Input: part model. Units: mm. Frame: model coordinates. A direction names the side the tool comes from. Round coordinates to 2 decimals unless told otherwise and drop trailing zeros. Loops run counter-clockwise (first coordinate to the right, second up) from the corner with the lowest first, then second, coordinate; pieces in that order, holes last.
(1) Cut plane A-A, the plane x = 0. Output: boundary loops of the cut face in (y, z).
(2) Cut plane B-B, the plane y = 0.75. Output: boundary loops of the cut face in (x, z).
(3) Access query for faces 1 (the face through (-1.245, 3.95, -3.002)), 2 (the face through (2, 2, 1)), 3 (the face through (-0.03, 0.27, -1.73)). Directions: +Z, -Z, +X, -X, +Y, -Y. A direction counts if a zero-diameter tool reaches every point of the face in a straight line with its end or side. Return the directions, or none.
(4) Draft query along Z for faces 4 (the face through (2, 3.2, 0)), 5 (the face through (0, 0, -2.3)), 6 (the face through (0.05, 0.13, -2.92)). Return one class per face: released by +Z, released by -Z, zero draft, split by the parting line, or undercut.
(5) Cut plane D-D, the plane y = 5.75. Output: boundary loops of the cut face in (x, z), and give its area (3 significant figures).
(6) Cut plane C-C, the plane z = 0. Output: boundary loops of the cut face in (x, y), and give its area (3 significant figures).
(7) First-contact query: pin 1 Ø1.5 at (y, z) = (1, 2) entering from +X; pin 2 Ø3.5 at (x, z) = (0, 0) entering from +Y; pin 3 Ø0.6 at (x, z) = (-2, 0.5) entering from -Y. Flat tips, straight axial feed; report the tip coordinate or a pass-through.
(8) Line query: line 1 (X direction, y = 6, z = 0); line 2 (Z direction, x = -0.75, y = 4); line 3 (X direction, y = 3.5, z = -0.5). Output: solid intervals per line, ascending.
Autodesk Inventor part; units mm, degrees
ref_plane "YZ Plane" through (0, 0, 0) normal (1, 0, 0) x (0, 1, 0)
ref_plane "XZ Plane" through (0, 0, 0) normal (0, 1, 0) x (-1, 0, 0)
ref_plane "XY Plane" through (0, 0, 0) normal (0, 0, 1) x (1, 0, 0)
sketch "__4" plane through (0, 0, 0) normal (1, 0, 0) x (0, 1, 0)
  line L0 (0, 0) -> (8, 0)
  line L1 (8, 0) -> (8, -2.79)
  line L2 (8, -2.79) -> (7.54, -3.25)
  line L3 (7.54, -3.25) -> (0.46, -3.25)
  line L4 (0.46, -3.25) -> (0, -2.79)
  line L5 (0, -2.79) -> (0, 0)
  line L6 (0, 0) -> (8, 0)
revolve "Revolution1" add sketch "__4" angle 360 about axis through (0, 0, 0) along (0, -1, 0)
sketch "__5" plane through (0, 0, 0) normal (1, 0, 0) x (0, 1, 0)
  line L0 (0, 0) -> (8, 0)
  line L1 (8, 0) -> (8, -2)
  line L2 (8, -2) -> (7.621, -1.621)
  line L3 (7.621, -1.621) -> (0.379, -1.621)
  line L4 (0.379, -1.621) -> (0, -2)
  line L5 (0, -2) -> (0, 0)
  line L6 (0, 0) -> (8, 0)
revolve "Revolution2" cut sketch "__5" angle 360 about axis through (0, 0, 0) along (0, -1, 0)
thread "Thread1"
sketch "__6" plane through (0, 0, 0) normal (1, 0, 0) x (0, 1, 0)
  line L0 (3.2, 1) -> (0, 1)
  line L1 (0, 1) -> (0, -1)
  line L2 (0, -1) -> (3.2, -1)
  line L3 (3.2, -1) -> (3.2, 1)
extrude "Extrusion1" cut sketch "__6" along normal mid plane 13
properties part number "105.040" material "Steel"
Reported:
1. outline: (0, -2.79) - (0.46, -3.25) - (7.54, -3.25) - (8, -2.79) - (8, -2) - (7.62, -1.62) - (0.38, -1.62) - (0, -2) - close; (0, 2) - (0.38, 1.62) - (7.62, 1.62) - (8, 2) - (8, 2.79) - (7.54, 3.25) - (0.46, 3.25) - (0, 2.79) - close
2. outline: (-3.09, -1) arc R3.25 ccw to (3.09, -1) - (1.28, -1) arc R1.62 cw to (-1.28, -1) - close; (-3.09, 1) - (-1.28, 1) arc R1.62 cw to (1.28, 1) - (3.09, 1) arc R3.25 ccw to start
3. face 1: +Y, -Y
3. face 2: +X, -X, -Y
3. face 3: -Y
4. face 4: undercut
4. face 5: zero draft
4. face 6: released by -Z
5. outline: circle Ø6.5 at (0, 0); hole circle Ø3.24 at (0, 0)
5. area: 24.9 mm2
6. outline: (-3.25, 3.2) - (-1.62, 3.2) - (-1.62, 7.62) - (-2, 8) - (-2.79, 8) - (-3.25, 7.54) - close; (1.62, 3.2) - (3.25, 3.2) - (3.25, 7.54) - (2.79, 8) - (2, 8) - (1.62, 7.62) - close
6. area: 15.3 mm2
7. pin 1: stops at x = 3
7. pin 2: stops at y = 7.75
7. pin 3: stops at y = 3.2
8. line 1: x = -3.25 to -1.62, 1.62 to 3.25
8. line 2: z = -3.16 to -1.44, 1.44 to 3.16
8. line 3: x = -3.21 to -1.54, 1.54 to 3.21
